Can you work these out from the drawing? Everything is in mm from the part's minimum corner. Round coordinates to 2 decimals unless told otherwise and drop trailing zeros. Loops run counter-clockwise (first coordinate to the right, second up) from the corner with the lowest first, then second, coordinate; pieces in that order, holes last. Notation, with made-up numbers: (-17, 21.5) -> (31, 21.5) arc R34 ccw to (31, 55.5) -> close; hole circle Ø6 at (25, 68). An arc over 180 degrees is marked (long way). One line per item, written item: value.
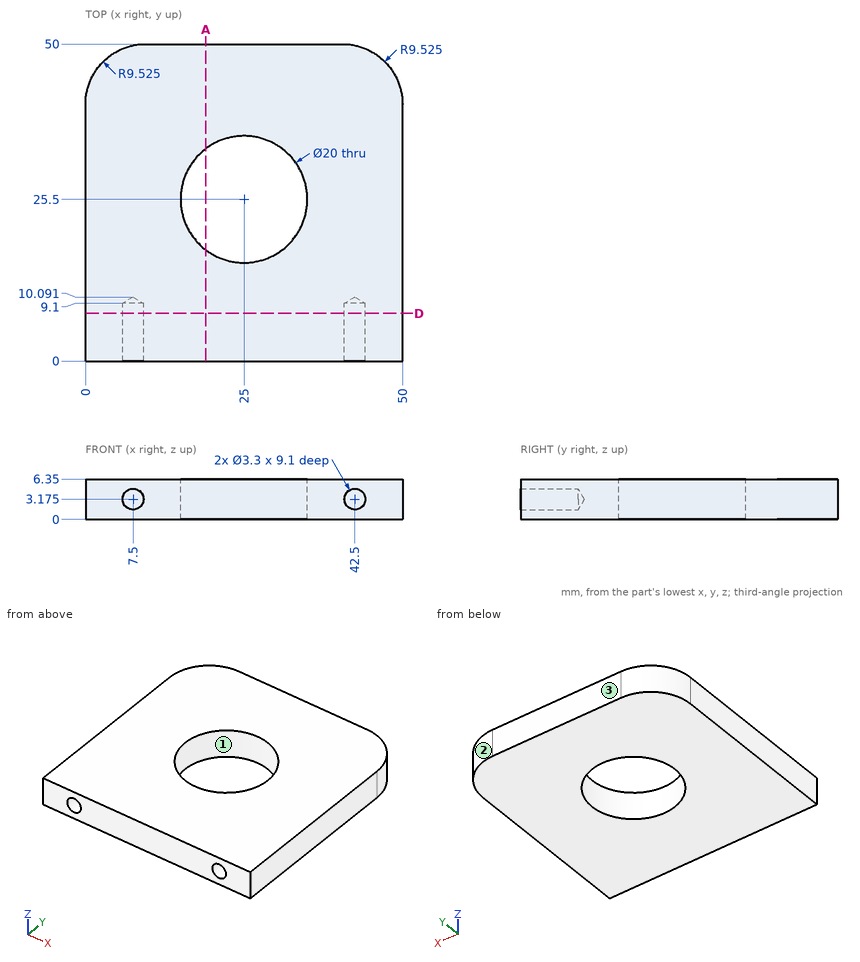
Item 1: If we mould it in two halves opening along X, with no side actions, what happens to the marked faces 1, 2 and 3? For each: released by +X, released by -X, zero draft, split by the parting line, or undercut.
Output:
face 1: undercut
face 2: released by +X
face 3: zero draft
Item 2: If we section it at A-A on x = 19: List the corners of the cut face in (y, z) for me, plus the area to 3 significant figures.
Output:
outline: (0, 0) -> (17.5, 0) -> (17.5, 6.35) -> (0, 6.35) -> close; (33.5, 0) -> (50, 0) -> (50, 6.35) -> (33.5, 6.35) -> close
area: 216 mm²
Item 3: Will this pin go through, and if not, where does the flat tip stop? pin 1 Ø3 at (x, z) = (42.5, 3.175) entering from +Y.
Output:
pin 1: stops at y = 49.99
Item 4: I need wall thicknesses on line 1 (Y direction, x = 25, z = 2); line 2 (Y direction, x = 21, z = 2.25) (1 decimal); line 3 (X direction, y = 26, z = 1.5). Which ranges of each line are inside material? Lowest first, please. Write a range as from..to.
Output:
line 1: y = 0..15.5, 35.5..50
line 2: y = 0..16.3, 34.7..50
line 3: x = 0..15.01, 34.99..50
Item 5: If we section it at D-D on y = 7.5: Count the separate pieces of the cut face and the enclosed holes in it.
Output:
separate pieces: 1
enclosed holes: 2
